Check sheet for the modelled part. Datum: model origin and axes. Units: mm. A direction names the side the tool comes from. Give positions to 0.01 mm unless a question says otherwise; leave off trailing zeros. Loops run counter-clockwise (first coordinate to the right, second up) from the corner with the lowest first, then second, coordinate; pieces in that order, holes last. Notation, with made-up numbers: (79, -27.5) -> (116, -27.5) arc R14 cw to (116, -5.5) -> close; hole circle Ø6 at (-3.5, 18). An arc over 180 degrees is marked (long way). Write each question's results on one line, items separated by ' | '. Start each with the question number.
Item 1: Cross-section at B-B on z = 7.25. Enter the section's corners in (x, y).
Item 2: Mould release check, pull along Y, two halves, no side actions. Record for faces 1 (the face through (51.17, 18.95, 3.13)), 2 (the face through (0, 13, 2)): pulls with the +Y half, pulls with the -Y half, needs draft (parallel to the pull), parting line crosses it, or undercut.
Item 3: Cross-section at A-A on x = 38.86. Enter the section's corners in (y, z), then the cut area to 3 significant figures.
Item 4: Scan lines: line 1 along Y through (x, z) = (62.74, 1.05); line 2 along Y through (x, z) = (50.8, 3.5); line 3 along X through (y, z) = (15.5, 7.25). Record each from-to range of solid material in increasing order.
Item 5: Access from +Z, -Z, +X, -X, +Y, -Y to the whole of each face (thin tool, end or side, straight path). Record for faces 3 (the face through (55.562, 13, 8)), 4 (the face through (58.738, 13, 7)), 5 (the face through (21, 13, 4.762)).
Item 6: Gauge pin test, flat ends, axial feed: pin 1 Ø1.9 at (x, y) = (38.86, 20.7) entering from -Z; pin 2 Ø4 at (x, y) = (50.8, 4.76) entering from +Z; pin 3 Ø2.5 at (x, y) = (94.74, 20.7) entering from +Z; pin 4 Ø4 at (y, z) = (13, 7) entering from -X. Record the tip position at first contact, or that the pin passes through.
Item 7: Cross-section at D-D on x = 50.8. Enter the section's corners in (y, z), then the cut area to 3 significant figures.
from build123d import *

# Parameters (mm, degrees)
SKETCH1_W                       = 101.6
SKETCH1_H                       = 25.4
BOSS_EXTRUDE1_DEPTH             = 9.525
SKETCH2_W                       = 9.525
SKETCH2_H                       = 3.175
SKETCH2_W_2                     = 42.8625
SKETCH2_H_2                     = 4.7625
CUT_EXTRUDE1_DEPTH              = 106.159144277
F_8_32_TAPPED_HOLE1_D           = 3.4544
F_45_0_082_DIAMETER_HOLE1_D     = 2.0828
F_45_0_082_DIAMETER_HOLE1_DEPTH = 9.652
F_45_0_082_DIAMETER_HOLE1_TIP   = 0.625736249


with BuildPart() as part:
    # Sketch1 → Boss-Extrude1 (new body)
    with BuildSketch(Plane.XY):
        with Locations((50.8, 12.7)):
            Rectangle(SKETCH1_W, SKETCH1_H)
    extrude(amount=BOSS_EXTRUDE1_DEPTH)

    # Sketch2 → Cut-Extrude1 (cut, through all)
    with BuildSketch(Plane(origin=(0, 25.4, 0), x_dir=(1, 0, 0), z_dir=(0, 1, 0))):
        with Locations((50.8, -7.9375)):
            Rectangle(SKETCH2_W, SKETCH2_H)
        with Locations((21.43125, -7.14375)):
            Rectangle(SKETCH2_W_2, SKETCH2_H_2)
        with Locations((80.16875, -7.14375)):
            Rectangle(SKETCH2_W_2, SKETCH2_H_2)
    extrude(amount=-CUT_EXTRUDE1_DEPTH, mode=Mode.SUBTRACT)

    # #8-32 Tapped Hole1 (through all)
    with Locations(Plane.XY.offset(6.35)):
        with Locations((50.8, 4.7625), (50.8, 20.6375)):
            Hole(F_8_32_TAPPED_HOLE1_D / 2)

    # #45 (0.082) Diameter Hole1
    with Locations(Plane(origin=(0, 0, 0), x_dir=(-1, 0, 0), z_dir=(0, 0, -1))):
        with Locations((-38.86, 20.7), (-6.86, 20.7), (-38.86, 4.7), (-6.86, 4.7), (-62.74, 4.7), (-94.74, 4.7), (-62.74, 20.7), (-94.74, 20.7)):
            Hole(F_45_0_082_DIAMETER_HOLE1_D / 2, depth=F_45_0_082_DIAMETER_HOLE1_DEPTH)
            with Locations((0, 0, -(F_45_0_082_DIAMETER_HOLE1_DEPTH + F_45_0_082_DIAMETER_HOLE1_TIP / 2))):  # 118° drill point
                Cone(0, F_45_0_082_DIAMETER_HOLE1_D / 2, F_45_0_082_DIAMETER_HOLE1_TIP, mode=Mode.SUBTRACT)


solid = part.part
Answer sheet:
1) outline: (42.86, 0) -> (46.04, 0) -> (46.04, 25.4) -> (42.86, 25.4) -> close; (55.56, 0) -> (58.74, 0) -> (58.74, 25.4) -> (55.56, 25.4) -> close
2) face 1: undercut | face 2: needs draft
3) outline: (0, 0) -> (3.66, 0) -> (3.66, 4.76) -> (0, 4.76) -> close; (5.74, 0) -> (19.66, 0) -> (19.66, 4.76) -> (5.74, 4.76) -> close; (21.74, 0) -> (25.4, 0) -> (25.4, 4.76) -> (21.74, 4.76) -> close | area: 101 mm²
4) line 1: y = 0 to 3.66, 5.74 to 19.66, 21.74 to 25.4 | line 2: y = 0 to 3.04, 6.49 to 18.91, 22.36 to 25.4 | line 3: x = 42.86 to 46.04, 55.56 to 58.74
5) face 3: +Z, +Y, -Y | face 4: +Z, +X, +Y, -Y | face 5: +Z, -X, +Y, -Y
6) pin 1: passes through | pin 2: stops at z = 6.35 | pin 3: stops at z = 4.76 | pin 4: stops at x = 42.86
7) outline: (0, 0) -> (3.04, 0) -> (3.04, 6.35) -> (0, 6.35) -> close; (6.49, 0) -> (18.91, 0) -> (18.91, 6.35) -> (6.49, 6.35) -> close; (22.36, 0) -> (25.4, 0) -> (25.4, 6.35) -> (22.36, 6.35) -> close | area: 117 mm²
